Read the model definition and answer for the solid it produces. Units are mm, in the model's axes. A direction names the side the tool comes from. Coordinates: 2 decimals unless noted, no trailing zeros. Loops run counter-clockwise (first coordinate to the right, second up) from the corner with the lowest first, then second, coordinate; pieces in that order, holes last. Notation, with made-up numbers: M 38,-28 L 76,-28 A29 ccw 76,4 Z; hole C -25.5,12 d4. An arc over 180 degrees is marked long. Put each result on its own line as item: value.
from build123d import *

# Parameters (mm, degrees)
F0_W      = 63.5
F0_H      = 72.263
F1_DEPTH  = 2.794
F2_W      = 2.794
F2_H      = 72.263
F3_DEPTH  = 16.256
F4_W      = 1.5875
F4_H      = 2.794
F5_DEPTH  = 16.256
F6_W      = 1.5875
F6_H      = 2.794
F7_DEPTH  = 16.256
F8_W      = 1.5875
F8_H      = 3.175
F9_DEPTH  = 2.794
F10_W     = 1.5875
F10_H     = 3.174931046
F11_DEPTH = 2.794


# Not quite as in the source:
# - a feature names something its author has since deleted; it is built from what else it names


with BuildPart() as f1:
    # F0 (on Top) → F1 (new body)
    with BuildSketch(Plane.XY):
        Rectangle(F0_W, F0_H)
    extrude(amount=-F1_DEPTH)

    # F2 (on face) → F3 (join)
    with BuildSketch(Plane.XY):
        with Locations((-30.353, 0)):
            Rectangle(F2_W, F2_H)
        with Locations((30.353, 0)):
            Rectangle(F2_W, F2_H)
    extrude(amount=F3_DEPTH)

    # F4 (on face) → F5 (cut, through all)
    with BuildSketch(Plane.XY.offset(16.256)):
        with Locations((-29.74975, 33.147)):
            Rectangle(F4_W, F4_H)
        with Locations((-29.74975, -33.147)):
            Rectangle(F4_W, F4_H)
    extrude(amount=-F5_DEPTH, mode=Mode.SUBTRACT)

    # F6 (on face) → F7 (cut, through all)
    with BuildSketch(Plane.XY.offset(16.256)):
        with Locations((29.74975, 33.147)):
            Rectangle(F6_W, F6_H)
        with Locations((29.74975, -33.147)):
            Rectangle(F6_W, F6_H)
    extrude(amount=-F7_DEPTH, mode=Mode.SUBTRACT)

    # F8 (on face) → F9 (cut, through all)
    with BuildSketch(Plane.YZ.offset(-28.956)):
        with Locations((21.81225, 14.6685)):
            Rectangle(F8_W, F8_H)
    extrude(amount=-F9_DEPTH, mode=Mode.SUBTRACT)

    # F10 (on face) → F11 (cut, through all)
    with BuildSketch(Plane(origin=(28.956, 0, 0), x_dir=(0, -1, 0), z_dir=(-1, 0, 0))):
        with Locations((-21.7913250594, 14.668534477)):
            Rectangle(F10_W, F10_H)
    extrude(amount=-F11_DEPTH, mode=Mode.SUBTRACT)


solid = f1.part
1) Given pin 1 Ø1.7 at (x, y) = (30, 22) entering from +Z; pin 2 Ø0.5 at (x, y) = (-30, 21.5) entering from +Z; pin 3 Ø3 at (x, y) = (-13.5, 15) entering from +Z, each flat-ended and moving along its own axis, determine where each tip first touches the part or whether it passes through.
Answer list:
pin 1: stops at z = 16.26
pin 2: stops at z = 13.08
pin 3: stops at z = 0
2) Straight lines are drawn through the part: line 1 (X direction, y = -12.5, z = 15.75); line 2 (X direction, y = 33.5, z = 6.25); line 3 (Z direction, x = 26, y = 17). For each, find the intervals that lie inside material, in ascending order. Write a range as [from, to].
Answer list:
line 1: x = [-31.75, -28.96], [28.96, 31.75]
line 2: x = [-31.75, -30.54], [30.54, 31.75]
line 3: z = [-2.79, 0]
3) Find section C-C, the plane y = -28. Write down the section's boundary in (x, z).
Answer list:
outline: M -31.75,-2.79 L 31.75,-2.79 L 31.75,16.26 L 28.96,16.26 L 28.96,0 L -28.96,0 L -28.96,16.26 L -31.75,16.26 Z
4) Find section B-B, the plane z = 7. Write down the section's boundary in (x, y), plus the area to 3 significant figures.
Answer list:
outline: M -31.75,-36.13 L -28.96,-36.13 L -28.96,-34.54 L -30.54,-34.54 L -30.54,-31.75 L -28.96,-31.75 L -28.96,31.75 L -30.54,31.75 L -30.54,34.54 L -28.96,34.54 L -28.96,36.13 L -31.75,36.13 Z; M 28.96,-36.13 L 31.75,-36.13 L 31.75,36.13 L 28.96,36.13 L 28.96,34.54 L 30.54,34.54 L 30.54,31.75 L 28.96,31.75 L 28.96,-31.75 L 30.54,-31.75 L 30.54,-34.54 L 28.96,-34.54 Z
area: 386 mm^2
5) Determine the mould class of faces 1 (the flat face through (30.543, -33, 8)), 2 (the flat face through (30, 29, 16.256)), 3 (the flat face through (30, 22.585, 15)) for opening direction Y: released by +Y, released by -Y, zero draft, split by the parting line, or undercut.
Answer list:
face 1: undercut
face 2: zero draft
face 3: undercut
6) Which of the six approach directions +Z, -Z, +X, -X, +Y, -Y give full straight-line access (tool end or side, diameter ignored) to faces 4 (the flat face through (28.956, 0, 8)), 5 (the flat face through (-30.543, 33, 8)), 6 (the flat face through (-31.75, -1, 7))?
Answer list:
face 4: +Z, +Y, -Y
face 5: +Z
face 6: +Z, -Z, -X, +Y, -Y
7) Find section A-A, the plane z = 14. Count the separate pieces of the cut face and the enclosed holes in it, plus the area to 3 significant figures.
Answer list:
separate pieces: 4
enclosed holes: 0
area: 377 mm^2
8) Find section D-D, the plane x = -25.5. Write down the section's boundary in (y, z), plus the area to 3 significant figures.
Answer list:
outline: M -36.13,-2.79 L 36.13,-2.79 L 36.13,0 L -36.13,0 Z
area: 202 mm^2
